from build123d import *

# Parameters (mm, degrees)
F0_W     = 6.604
F0_H     = 6.604
F1_DEPTH = 10.033
F2_R     = 1.651
F3_DEPTH = 2.032
F7_R     = 0.8136293968
F8_R     = 1.5330256121
F9_R     = 0.551182731


with BuildPart() as f1:
    # F0 (on Top) → F1 (new body)
    with BuildSketch(Plane.XY):
        Rectangle(F0_W, F0_H)
    extrude(amount=F1_DEPTH)

    # F2 (on face) → F3 (join)
    with BuildSketch(Plane(origin=(0, 0, 0), x_dir=(1, 0, 0), z_dir=(0, 0, -1))):
        Circle(F2_R)
    extrude(amount=F3_DEPTH)

    # F5 (on mid) → F6 (revolve)
    with BuildSketch(Plane.XZ):
        Polygon((2.7225008234, -1.9854432903), (1.6116809566, -1.9854432903), (0, -1.9854432903), (0, -10.8945909888), (0.4067335685, -10.8945909888), (2.7225008234, -8.0052432903), align=None)
    revolve(axis=Axis((0, 0, -6.4400171395), (0, 0, 1)))

    # F7
    f7_edges = [f1.edges().sort_by_distance(p)[0] for p in [
        (-0.406734, 0, -10.894591),
    ]]
    fillet(f7_edges, radius=F7_R)

    # F8
    f8_edges = [f1.edges().sort_by_distance(p)[0] for p in [
        (-3.302, -3.302, 5.0165),
        (3.302, -3.302, 5.0165),
        (3.302, 3.302, 5.0165),
        (-3.302, 3.302, 5.0165),
    ]]
    fillet(f8_edges, radius=F8_R)

    # F9
    f9_edges = [f1.edges().sort_by_distance(p)[0] for p in [
        (-2.722501, 0, -8.005243),
    ]]
    fillet(f9_edges, radius=F9_R)


solid = f1.part
Input: part model. Units: mm. Frame: model coordinates. A direction names the side the tool comes from. Round coordinates to 2 decimals unless told otherwise and drop trailing zeros. Loops run counter-clockwise (first coordinate to the right, second up) from the corner with the lowest first, then second, coordinate; pieces in that order, holes last. Notation, with made-up numbers: (-8, -7) -> (40, -7) arc R21 ccw to (40, 11) -> close; hole circle Ø4 at (81.25, -25.75). An arc over 180 degrees is marked (long way). Answer as a JSON object with one key per item and string values. Group by question number.
1) Reachability of faces 1 (the cylindrical face through (2.597, 0.818, -4.858)), 2 (the flat face through (-2, 1, 0)), 3 (the flat face through (-3.302, 0, 5)) from +Z, -Z, +X, -X, +Y, -Y: full face, straight path, thin tool, end or side. Return the list, or none.
2) Section query A-A on z = 7. Output: boundary loops of the cut face in (x, y).
3) Ray query, L1, parallel to X at y = 0, z = -1; L2, parallel to X at y = 0, z = -2.25; L3, parallel to Z at x = -0.25, y = -2.25. Return the intervals inside material, ascending.
4) Pin query (flat end, axial travel): pin 1 (1.5 mm diameter, centred on x = -2.5, z = -6, fed in from -Y); pin 2 (3 mm diameter, centred on x = 1, z = -7, fed in from -Y); pin 3 (1 mm diameter, centred on y = -2.5, z = -4, fed in from +X). Return the tip coordinate at first contact, or that it passes through.
5) Section query B-B on y = -3. Output: boundary loops of the cut face in (x, z), plus the area to 3 significant figures.
6) Section query C-C on z = -6.5. Output: boundary loops of the cut face in (x, y) (1 decimal), plus the area to 3 significant figures.
7) Draft query along Z for faces 4 (the cylindrical face through (2.841, -2.865, 5.087)), 5 (the flat face through (0, -2, -1.985)), 6 (the flat face through (0, 0, 10.033)). Return one class per face: +Z half, -Z half, draft (parallel to the pull), parting line (faces both ways), or undercut.
Reply:
{
 "1": {"face 1": "-Z", "face 2": "none", "face 3": "+Z, -Z, -X, +Y, -Y"},
 "2": {"outline": "(-3.3, -1.77) arc R1.53 ccw to (-1.77, -3.3) -> (1.77, -3.3) arc R1.53 ccw to (3.3, -1.77) -> (3.3, 1.77) arc R1.53 ccw to (1.77, 3.3) -> (-1.77, 3.3) arc R1.53 ccw to (-3.3, 1.77) -> close"},
 "3": {"L1": "x = -1.65 to 1.65", "L2": "x = -2.72 to 2.72", "L3": "z = -8.58 to -1.99, 0 to 10.03"},
 "4": {"pin 1": "stops at y = -2.09", "pin 2": "stops at y = -2.72", "pin 3": "stops at x = 1.85"},
 "5": {"outline": "(-2.68, 0) -> (2.68, 0) -> (2.68, 10.03) -> (-2.68, 10.03) -> close", "area": "53.8 mm2"},
 "6": {"outline": "circle Ø5.4 at (0, 0)", "area": "23.3 mm2"},
 "7": {"face 4": "draft", "face 5": "undercut", "face 6": "+Z half"}
}
